Could you check a few things on this model? Use its own coordinates, in mm. A direction names the side the tool comes from. Give positions to 0.01 mm unless a question says otherwise; leave off trailing zeros. Loops run counter-clockwise (first coordinate to the right, second up) from the corner with the lowest first, then second, coordinate; pieces in that order, holes last. Notation, with made-up numbers: M 54.25,-3 L 79.25,-3 A8 cw 79.25,7 Z; hole C 71,-10 d4. An arc over 180 degrees is marked long. Use a Markdown table: item, result. Add a question column.
1) Suppose I cut it at D-D on z = 654. List the corners of the cut face in (x, y) for me.
2) Which directions (+Z, -Z, +X, -X, +Y, -Y) give clear straight access to the entire face, cutting with the end or side of a thin tool? Please do faces 1 (the flat face through (-387.68, 787.85, 613.35)), 2 (the flat face through (-387.675, 237.555, 113.826)), 3 (the flat face through (-387.675, 959.174, 507.519)), 4 (the flat face through (-375, 659, 346)).
3) Will these pins go through, and if not, where does the flat tip stop? pin 1 Ø8 at (x, y) = (-390, 314) entering from -Z (3 decimals); pin 2 Ø4 at (x, z) = (-383, 111) entering from -Y; pin 3 Ø4 at (x, y) = (-387, 283) entering from +Z.
4) Suppose I cut it at C-C on y = 349. List the corners of the cut face in (x, z) for me.
5) We'd pull the mould along Y, two halves only. Please class faces 5 (the flat face through (-388, 112, 0)), 6 (the cylindrical face through (-387.32, 201.25, 7.04)), 7 (the cylindrical face through (-387.325, 711.417, 6.656)), 8 (the flat face through (-387.68, 1005.7, 841.75)): +Y half, -Y half, draft (parallel to the pull), parting line (faces both ways), or undercut.
6) If I drill on line 1 along Y through (x, z) = (-396.5, 131); line 2 along Z through (x, y) = (-394, 203.5); line 3 along Z through (x, y) = (-398.25, 710.5), over which ranges is the centre line in solid material (lowest first)? Write a range as [from, to].
7) Suppose I cut it at B-B on x = -392.25. List the corners of the cut face in (y, z) for me, and give its area (3 significant figures).
8) Suppose I cut it at A-A on z = 414. List the corners of the cut face in (x, y) for me, and give its area (3 significant figures).
```python
from build123d import *

# Parameters (mm, degrees)
F2_DEPTH = 25
F3_R     = 35
F4_R     = 35


with BuildPart() as f2:
    # F1 (on offset) → F2 (new body)
    with BuildSketch(Plane.YZ.offset(-400)):
        Polygon((129.409523, 482.962913), (0, 0), (207.055236, 0), (270.830879, 238.013939), (660.668727, 133.557202), (707.055236, 0), (918.77469, 0), (834.995909, 241.21797), (1095.501241, 799.873458), (914.239684, 884.397111), (660.668727, 340.612438), align=None)
    extrude(amount=F2_DEPTH)

    # F3
    f3_edges = [f2.edges().sort_by_distance(p)[0] for p in [
        (-387.5, 914.239684, 884.397111),
        (-387.5, 1095.501241, 799.873458),
        (-387.5, 660.668727, 340.612438),
        (-387.5, 129.409523, 482.962913),
        (-387.5, 707.055236, 0),
        (-387.5, 0, 0),
        (-387.5, 918.77469, 0),
        (-387.5, 207.055236, 0),
        (-387.5, 270.830879, 238.013939),
        (-387.5, 660.668727, 133.557202),
    ]]
    fillet(f3_edges, radius=F3_R)

    # F4
    f4_edges = [f2.edges().sort_by_distance(p)[0] for p in [
        (-387.5, 834.995909, 241.21797),
    ]]
    fillet(f4_edges, radius=F4_R)


solid = f2.part
```
Answer block:
| question | item | result |
|---|---|---|
| 1 | outline | M -400,806.8 L -375,806.8 L -375,1027.48 L -400,1027.48 Z |
| 2 | face 1 | +Z, +X, -X |
| 2 | face 2 | -Z, +X, -X |
| 2 | face 3 | +X, -X, +Y |
| 2 | face 4 | +Z, -Z, +X, +Y, -Y |
| 3 | pin 1 | stops at z = 225.375 |
| 3 | pin 2 | stops at y = 29.21 |
| 3 | pin 3 | stops at z = 442.34 |
| 4 | outline | M -400,217.07 L -375,217.07 L -375,424.12 L -400,424.12 Z |
| 5 | face 5 | draft |
| 5 | face 6 | undercut |
| 5 | face 7 | undercut |
| 5 | face 8 | +Y half |
| 6 | line 1 | y = [35.1, 242.16], [656.61, 873.28] |
| 6 | line 2 | z = [8.88, 463.11] |
| 6 | line 3 | z = [7.34, 447.48] |
| 7 | outline | M 11.81,44.06 A35 ccw 45.61,0 L 180.2,0 A35 ccw 214.01,25.94 L 261.77,204.21 A35 cw 304.64,228.96 L 642.75,138.36 A35 cw 666.75,116.03 L 698.89,23.52 A35 ccw 731.95,0 L 869.57,0 A35 ccw 902.63,46.48 L 839.65,227.81 A35 cw 841,254.08 L 1080.71,768.15 A35 ccw 1063.78,814.67 L 945.96,869.61 A35 ccw 899.45,852.68 L 673.08,367.23 A35 cw 632.3,348.21 L 163.22,473.9 A35 ccw 120.35,449.16 Z |
| 7 | area | 348,000 mm^2 |
| 8 | outline | M -400,110.93 L -375,110.93 L -375,386.78 L -400,386.78 Z; M -400,694.89 L -375,694.89 L -375,915.57 L -400,915.57 Z |
| 8 | area | 12,400 mm^2 |
